The listing builds one solid part. Answer for the finished solid, in the listing's coordinates (mm). Coordinates: 2 decimals unless noted, no trailing zeros. Order: outer loops, then holes, each group sorted by start corner. A loop starts at its lowest first (then second) coordinate and runs counter-clockwise, first axis right, second up. Notation, with made-up numbers: (20, 24.5) -> (27, 24.5) arc R18 cw to (27, 42.5) -> close; hole circle Ø10 at (28.5, 70.5). An arc over 180 degrees is marked (long way). Write item = value, one per line. Start each with the question number.
Autodesk Inventor part; units mm, degrees
ref_plane "Work Plane1" through (0, 0, -7.5) normal (-1, 0, 0) x (0, 0, 1)
ref_plane "YZ Plane" through (0, 0, 0) normal (1, 0, 0) x (0, 1, 0)
ref_plane "XZ Plane" through (0, 0, 0) normal (0, 1, 0) x (-1, 0, 0)
sketch "Sketch1" plane through (0, 0, 0) normal (0, 1, 0) x (-1, 0, 0)
  line L0 (-49.75, 7.5) -> (49.75, 7.5)
  line L1 (49.75, 7.5) -> (49.75, -7.5)
  line L2 (49.75, -7.5) -> (-49.75, -7.5)
  line L3 (-49.75, -7.5) -> (-49.75, 7.5)
  line L4 (-49.75, 7.5) -> (49.75, -7.5) construction
  line L5 (49.75, 7.5) -> (-49.75, -7.5) construction
  point P0 (0, 0)
  dimension "d0" = 15
  dimension "d1" = 99.5
extrude "Extrusion1" add sketch "Sketch1" along normal blind 2
sketch "Sketch2" plane through (0, 2, 0) normal (0, 1, 0) x (1, 0, 0)
  line L0 (49.75, 7.5) -> (-49.75, 7.5)
  line L1 (49.75, -7.5) -> (49.75, 7.5)
  point P0 (0, 0)
  point P1 (23.75, 2.8)
  dimension "d11" = 4.7
  dimension "d12" = 26
hole "Hole1" at (23.75, 2, -2.8) direction (0, -1, 0) diameter 5.1 end through all
sketch "Sketch3" plane through (0, 0, 0) normal (0, -1, 0) x (1, 0, 0)
  line L0 (26.3, -0.25) -> (21.2, -0.25)
  line L1 (21.2, -0.25) -> (21.2, -5.35)
  line L2 (21.2, -5.35) -> (26.3, -5.35)
  line L3 (26.3, -5.35) -> (26.3, -0.25)
  circle A0 centre (23.75, -2.8) radius 2.55
  line L4 (26.3, -0.25) -> (21.2, -5.35) construction
  line L5 (21.2, -0.25) -> (26.3, -5.35) construction
  line L6 (25.3, -5.35) -> (25.3, -0.25)
  line L7 (22.2, -5.35) -> (22.2, -0.25)
  point P0 (0, 0)
  point P1 (22.2, -4.8248)
  point P2 (22.2, -0.7752)
  point P3 (25.3, -0.7752)
  point P4 (25.3, -4.8248)
  dimension "d13" = 5.1
  dimension "d14" = 5.1
  dimension "d15" = 1
  dimension "d16" = 1
extrude "Extrusion2" add sketch "Sketch3" against normal blind 1.25 contours A0 L6 | L7 A0
fillet "Fillet1" radius 0.2 2 edges at (25.3, 0, -2.8) (22.2, 0, -2.8)
ref_plane "Work Plane1" through (0, 0, -7.5) normal (-1, 0, 0) x (0, 0, 1)
mirror "Mirror1" about plane through (0, 0, -7.5) normal (-1, 0, 0) of "Hole1", "Extrusion2", "Fillet1"
sketch "Sketch4" plane through (-49.75, 0, -7.5) normal (-1, 0, 0) x (0, 0, 1)
  line L0 (0, 0) -> (15, 0)
  line L1 (15, 0) -> (8.8446, 2)
  line L2 (0, 2) -> (15, 2)
  line L3 (8.8446, 0) -> (15, 0)
  line L4 (8.8446, 2) -> (8.8446, 0)
  line L5 (15, 0) -> (15, 2)
  line L6 (8.8446, 2) -> (15, 2)
  line L7 (15, 2) -> (15, 0)
  point P0 (7.5, 0)
  dimension "d21" = 18
extrude "Extrusion3" cut sketch "Sketch4" against normal through all contours L1 L2 L5
fillet "Fillet2" radius 2 1 edges at (0, 2, 1.3446)
properties part number "Bladev2" material "Stainless Steel"
Item 1: Section C-C, the plane y = 0.65 is taken. Give the vertices of the cut face in (x, z).
Item 2: Consider probe 1 along X at (y, z) = (1.2, -4.25); probe 2 along X at (y, z) = (1.3, -2.8); probe 3 along Y at (x, z) = (-7, 4.5). Determine where each line is inside the solid, lowest interval first.
Item 3: This flat-tipped pin is pushed along its axis until it touches: pin 1 (0.5 mm diameter, centred on x = 21.5, z = -3, fed in from +Y). Where does it stop, or does it pass through?
Item 4: For a pull along Z with two mould halves and no side action, classify faces 1 (the flat face through (-49.75, 1, -2)), 2 (the flat face through (-1, 1, -7.5)), 3 (the cylindrical face through (24.727, 1.208, -0.444)), 4 (the cylindrical face through (-22.773, 1.208, -0.444)) as pulls with the +Z half, pulls with the -Z half, needs draft (parallel to the pull), parting line crosses it, or undercut.
Item 5: Section D-D, the plane x = 8 is taken. Give the vertices of the cut face in (y, z).
Item 6: Section A-A, the plane z = -2.8 is taken. Give the vertices of the cut face in (x, y).
Item 7: Section B-B, the plane x = 23.75 is taken. Give the vertices of the cut face in (y, z).
A:
q1.outline = (-49.75, -7.5) -> (49.75, -7.5) -> (49.75, 5.5) -> (-49.75, 5.5) -> close; hole (-25.3, -4.82) arc R2.55 ccw to (-22.2, -4.82) -> (-22.2, -0.78) arc R2.55 ccw to (-25.3, -0.78) -> close; hole (22.2, -4.82) arc R2.55 ccw to (25.3, -4.82) -> (25.3, -0.78) arc R2.55 ccw to (22.2, -0.78) -> close
q2.probe_1 = -49.75 to -25.3, -22.2 to 22.2, 25.3 to 49.75
q2.probe_2 = -49.75 to -26.3, -21.2 to 21.2, 26.3 to 49.75
q2.probe_3 = 0 to 0.97
q3.pin_1 = 1.25
q4.face_1 = needs draft
q4.face_2 = pulls with the -Z half
q4.face_3 = undercut
q4.face_4 = undercut
q5.outline = (0, -7.5) -> (2, -7.5) -> (2, 1.03) arc R2 ccw to (1.9, 1.65) -> (0, 7.5) -> close
q6.outline = (-49.75, 0) -> (-25.5, 0) arc R0.2 ccw to (-25.3, 0.2) -> (-25.3, 1.25) -> (-26.3, 1.25) -> (-26.3, 2) -> (-49.75, 2) -> close; (-22.2, 0.2) arc R0.2 ccw to (-22, 0) -> (22, 0) arc R0.2 ccw to (22.2, 0.2) -> (22.2, 1.25) -> (21.2, 1.25) -> (21.2, 2) -> (-21.2, 2) -> (-21.2, 1.25) -> (-22.2, 1.25) -> close; (25.3, 0.2) arc R0.2 ccw to (25.5, 0) -> (49.75, 0) -> (49.75, 2) -> (26.3, 2) -> (26.3, 1.25) -> (25.3, 1.25) -> close
q7.outline = (0, -7.5) -> (2, -7.5) -> (2, -5.35) -> (0, -5.35) -> close; (0, -0.25) -> (2, -0.25) -> (2, 1.03) arc R2 ccw to (1.9, 1.65) -> (0, 7.5) -> close
